For this review, take the finished solid that the model builds, in its own axes (mm). A direction names the side the tool comes from. Coordinates: 2 decimals unless noted, no trailing zeros. Order: outer loops, then holes, each group sorted by start corner. A loop starts at its lowest first (then second) coordinate and runs counter-clockwise, first axis right, second up.
from build123d import *
from OCP.BRepFilletAPI import BRepFilletAPI_MakeChamfer

# Parameters (mm, degrees)
SKETCH1_W           = 135.29
SKETCH1_H           = 128
BOSS_EXTRUDE1_DEPTH = 5
SKETCH2_W           = 129.29
SKETCH2_H           = 122
BOSS_EXTRUDE2_DEPTH = 3
FILLET4_R           = 5
FILLET5_R           = 5
FILLET6_R           = 2
CUT_EXTRUDE1_REACH  = 95.466
SKETCH3_W           = 135.29
SKETCH3_H           = 4.25
SKETCH4_W           = 123.29
SKETCH4_H           = 117.75
CUT_EXTRUDE2_DEPTH  = 3
FILLET7_R           = 2
SKETCH5_W           = 43.25
SKETCH5_H           = 69.75
CUT_EXTRUDE3_DEPTH  = 3
SKETCH6_W           = 43.25
SKETCH6_H           = 34
CUT_EXTRUDE4_DEPTH  = 2
FILLET9_R           = 3
CHAMFER1_SIZE       = 0.75
CHAMFER1_SIZE2      = 1.299038106
CHAMFER2_SIZE       = 0.75
CHAMFER2_SIZE_2     = 1.299038106
SKETCH7_W           = 26
SKETCH7_H           = 3
CUT_EXTRUDE5_DEPTH  = 3
CHAMFER3_SIZE       = 0.75
CHAMFER3_SIZE2      = 1.299038106


# Some blends are built 0.0001 mm under size
with BuildPart() as part:
    # Sketch1 → Boss-Extrude1 (new body)
    with BuildSketch(Plane(origin=(0, 0, 0), x_dir=(1, 0, 0), z_dir=(0, 1, 0))):
        Rectangle(SKETCH1_W, SKETCH1_H)
    extrude(amount=BOSS_EXTRUDE1_DEPTH)

    # Sketch2 → Boss-Extrude2 (add)
    with BuildSketch(Plane.XZ):
        Rectangle(SKETCH2_W, SKETCH2_H)
    extrude(amount=BOSS_EXTRUDE2_DEPTH)

    # Fillet4
    fillet4_edges = [part.edges().sort_by_distance(p)[0] for p in [
        (-67.645, 2.5, -64),
        (67.645, 2.5, -64),
        (67.645, 2.5, 64),
        (-67.645, 2.5, 64),
    ]]
    fillet(fillet4_edges, radius=FILLET4_R)

    # Fillet5
    fillet5_edges = [part.edges().sort_by_distance(p)[0] for p in [
        (-66.180533906, 5, -62.535533906),
        (-67.645, 5, 0),
        (-66.180533906, 5, 62.535533906),
        (0, 5, 64),
        (66.180533906, 5, 62.535533906),
        (67.645, 5, 0),
        (66.180533906, 5, -62.535533906),
        (0, 5, -64),
    ]]
    fillet(fillet5_edges, radius=FILLET5_R - 0.0001)  # a hair under: the kernel refuses the full size

    # Fillet6
    fillet6_edges = [part.edges().sort_by_distance(p)[0] for p in [
        (-64.645, -1.5, 61),
        (-64.645, -1.5, -61),
        (64.645, -1.5, -61),
        (64.645, -1.5, 61),
    ]]
    fillet(fillet6_edges, radius=FILLET6_R)

    # Cut-Extrude1: up to this face of the body (flat: up to its plane)
    cut_extrude1_end = Plane(part.part.faces().sort_by_distance((0, -3, 0))[0])
    # Sketch3 → Cut-Extrude1 (cut, up to the picked face)
    with BuildSketch(Plane(origin=(0, 5, 0), x_dir=(1, 0, 0), z_dir=(0, 1, 0)), mode=Mode.PRIVATE) as cut_extrude1_sk1:
        with Locations((0, 61.875)):
            Rectangle(SKETCH3_W, SKETCH3_H)
    cut_extrude1_tool1 = split(extrude(cut_extrude1_sk1.sketch, amount=-CUT_EXTRUDE1_REACH, mode=Mode.PRIVATE), bisect_by=cut_extrude1_end, keep=Keep.BOTH, mode=Mode.PRIVATE)
    add(cut_extrude1_tool1.solids().sort_by(Axis((0, 5, -61.875), (0, -1, 0)))[0], mode=Mode.SUBTRACT)

    # Sketch4 → Cut-Extrude2 (cut)
    with BuildSketch(Plane.XZ.offset(3)):
        with Locations((0, -0.875)):
            Rectangle(SKETCH4_W, SKETCH4_H)
    extrude(amount=-CUT_EXTRUDE2_DEPTH, mode=Mode.SUBTRACT)

    # Fillet7
    fillet7_edges = [part.edges().sort_by_distance(p)[0] for p in [
        (-61.645, -1.5, 58),
        (61.645, -1.5, 58),
    ]]
    fillet(fillet7_edges, radius=FILLET7_R)

    # Sketch5 → Cut-Extrude3 (cut)
    with BuildSketch(Plane(origin=(0, 5, 0), x_dir=(1, 0, 0), z_dir=(0, 1, 0))):
        with Locations((22.77, -29.125)):
            Rectangle(SKETCH5_W, SKETCH5_H)
    extrude(amount=-CUT_EXTRUDE3_DEPTH, mode=Mode.SUBTRACT)

    # Sketch6 → Cut-Extrude4 (cut)
    with BuildSketch(Plane(origin=(0, 2, 0), x_dir=(1, 0, 0), z_dir=(0, 1, 0))):
        with Locations((22.77, -11.25)):
            Rectangle(SKETCH6_W, SKETCH6_H)
    extrude(amount=-CUT_EXTRUDE4_DEPTH, mode=Mode.SUBTRACT)

    # Fillet9
    fillet9_edges = [part.edges().sort_by_distance(p)[0] for p in [
        (1.145, 2.5, -5.75),
        (44.395, 2.5, -5.75),
        (44.395, 1, 28.25),
        (1.145, 1, 28.25),
    ]]
    fillet(fillet9_edges, radius=FILLET9_R)

    # Chamfer1: one chamfer whose edges measure the first distance from different faces: ONE call of the kernel's chamfer builder (chamfer() names one face for all edges)
    chamfer1_edges_1 = [part.edges().sort_by_distance(p)[0] for p in [
        (44.395, 4.183298538, 61.738685401),
        (1.145, 4.183298538, 61.738685401),
    ]]
    chamfer1_side_1 = [part.faces().sort_by_distance(p)[0] for p in [
        (0, 3.535563195, 62.535563195),
    ]]
    chamfer1_edges_2 = [part.edges().sort_by_distance(p)[0] for p in [
        (44.395, 5, 28.12505),
        (1.145, 5, 28.12505),
        (22.77, 5, -5.75),
        (43.516320344, 5, -4.871320344),
        (2.023679656, 5, -4.871320344),
    ]]
    chamfer1_side_2 = [part.faces().sort_by_distance(p)[0] for p in [
        (-5.311957969, 5, -6.221509605),
    ]]
    chamfer1 = BRepFilletAPI_MakeChamfer(part.part.solid().wrapped)
    for e in chamfer1_edges_1:
        chamfer1.Add(CHAMFER1_SIZE, CHAMFER1_SIZE2, e.wrapped, chamfer1_side_1[0].wrapped)  # the first distance lies on this face
    for e in chamfer1_edges_2:
        chamfer1.Add(CHAMFER1_SIZE, CHAMFER1_SIZE2, e.wrapped, chamfer1_side_2[0].wrapped)  # the first distance lies on this face
    add(Compound.cast(chamfer1.Shape()), mode=Mode.REPLACE)

    # Chamfer2
    # the kernel refuses this chamfer: 1.299038106, 0.75 mm, written as the material it takes off along each edge
    with BuildSketch(Plane(origin=(41.395, 2, 28.25), x_dir=(0, 0.05789386240267144, 0.9983227437537926), z_dir=(-1, 0, 0))) as chamfer2_piece_1:
        Polygon((CHAMFER2_SIZE * 0.998322743754, -CHAMFER2_SIZE * 0.0578938624027), (-CHAMFER2_SIZE_2 * 0.0578938623883, -CHAMFER2_SIZE_2 * 0.998322743505), (0, 0), align=None)
    extrude(amount=37.25, mode=Mode.SUBTRACT)
    with BuildSketch(Plane(origin=(4.145, 2, 25.25), x_dir=(-0.43506037057501545, 0, -0.9004012849586179), z_dir=(0.9004012849586179, 0, -0.43506037057501545))) as chamfer2_piece_2_section:
        Polygon((3 + CHAMFER2_SIZE, 0), (3, -CHAMFER2_SIZE_2), (3, 0), align=None)
    chamfer2_piece_2 = revolve(axis=Axis((4.145, 2, 25.25), (0, 1, 0)), revolution_arc=154.210864587, mode=Mode.PRIVATE)
    chamfer2_piece_2 = split(chamfer2_piece_2, bisect_by=Plane(origin=(1.145, 1.523753347, 27.427166172), z_dir=(1, 0, 0)), keep=Keep.TOP, mode=Mode.PRIVATE)
    add(chamfer2_piece_2, mode=Mode.SUBTRACT)
    with BuildSketch(Plane(origin=(41.395, 2, 25.25), x_dir=(0, 0, 1), z_dir=(-1, 0, 0))) as chamfer2_piece_3_section:
        Polygon((3 + CHAMFER2_SIZE, 0), (3, -CHAMFER2_SIZE_2), (3, 0), align=None)
    chamfer2_piece_3 = revolve(axis=Axis((41.395, 2, 25.25), (0, 1, 0)), revolution_arc=154.210864587, mode=Mode.PRIVATE)
    chamfer2_piece_3 = split(chamfer2_piece_3, bisect_by=Plane(origin=(44.395, 1.633451558, 28.466921633), z_dir=(-1, 0, 0)), keep=Keep.TOP, mode=Mode.PRIVATE)
    add(chamfer2_piece_3, mode=Mode.SUBTRACT)

    # Sketch7 → Cut-Extrude5 (cut)
    with BuildSketch(Plane(origin=(64.645, 0, 0), x_dir=(0, 0, -1), z_dir=(1, 0, 0))):
        with Locations((19, -1.5)):
            Rectangle(SKETCH7_W, SKETCH7_H)
    extrude(amount=-CUT_EXTRUDE5_DEPTH, mode=Mode.SUBTRACT)

    # Chamfer3: one chamfer whose edges measure the first distance from different faces: ONE call of the kernel's chamfer builder (chamfer() names one face for all edges)
    chamfer3_edges_1 = [part.edges().sort_by_distance(p)[0] for p in [
        (64.645, -1.5, -6),
    ]]
    chamfer3_side_1 = [part.faces().sort_by_distance(p)[0] for p in [
        (64.645, -1.5, 26.5),
    ]]
    chamfer3_edges_2 = [part.edges().sort_by_distance(p)[0] for p in [
        (64.645, -1.5, -32),
    ]]
    chamfer3_side_2 = [part.faces().sort_by_distance(p)[0] for p in [
        (64.645, -1.5, -45.5),
    ]]
    chamfer3 = BRepFilletAPI_MakeChamfer(part.part.solid().wrapped)
    for e in chamfer3_edges_1:
        chamfer3.Add(CHAMFER3_SIZE, CHAMFER3_SIZE2, e.wrapped, chamfer3_side_1[0].wrapped)  # the first distance lies on this face
    for e in chamfer3_edges_2:
        chamfer3.Add(CHAMFER3_SIZE, CHAMFER3_SIZE2, e.wrapped, chamfer3_side_2[0].wrapped)  # the first distance lies on this face
    add(Compound.cast(chamfer3.Shape()), mode=Mode.REPLACE)


solid = part.part
1. Clearance check with flat-ended pins moving along their axes: pin 1 Ø4 at (x, z) = (-12, -1) entering from -Y; pin 2 Ø1.5 at (y, z) = (-1.5, 12.5) entering from -X (3 decimals); pin 3 Ø1.5 at (y, z) = (-1, -40) entering from +X (3 decimals). State where each tip first meets the part, or that it passes through.
Answer below:
pin 1: stops at y = 0
pin 2: stops at x = -64.645
pin 3: stops at x = 64.645
2. Machinability: for faces 1 (the face through (61.645, -2, -46)), 2 (the face through (64.645, -1, 26)), 3 (the face through (22, 2, 45)), which of the approach directions +Z, -Z, +X, -X, +Y, -Y give a long, thin tool a straight path to every point of the face, cutting with its end or side? Answer none if there is none.
Answer below:
face 1: -Z, -Y
face 2: +Z, -Z, +X, -Y
face 3: +Z, +Y
3. Take a section at B-B, the plane y = -1.5. Give the boundary of the cut face in (x, z) (3 decimals), plus the area to 3 significant figures.
Answer below:
outline: (-64.645, -59) arc R2 ccw to (-64.499, -59.75) - (-61.645, -59.75) - (-61.645, 56) arc R2 cw to (-59.645, 58) - (59.645, 58) arc R2 cw to (61.645, 56) - (61.645, -6) - (63.346, -6) - (64.645, -5.25) - (64.645, 59) arc R2 ccw to (62.645, 61) - (-62.645, 61) arc R2 ccw to (-64.645, 59) - close; (61.645, -59.75) - (64.499, -59.75) arc R2 ccw to (64.645, -59) - (64.645, -32.75) - (63.346, -32) - (61.645, -32) - close
area: 1,020 mm2
4. The part is to be moulded in two halves that separate along Z. For faces 4 (the face through (44.395, 2, 23)), 5 (the face through (43.744, 4.197, -5.048)), 6 (the face through (-64.645, -1, -1)), 7 (the face through (43.54, 0.35, 27.35)), say which applies: +Z half, -Z half, draft (parallel to the pull), parting line (faces both ways), or undercut.
Answer below:
face 4: undercut
face 5: +Z half
face 6: draft
face 7: undercut
5. To check wall thickness, follow L1, parallel to X at y = -2.25, z = 36 (3 decimals); L2, parallel to Y at x = 60, z = -53.5; L3, parallel to Y at x = 2, z = 39.5. State the ranges of each line that lie inside material, in increasing order.
Answer below:
L1: x = -64.645 to -61.645, 61.645 to 64.645
L2: y = 0 to 5
L3: y = 0 to 2
